Can you work these out from the drawing? Everything is in mm from the part's minimum corner. Coordinates: 2 decimals unless noted, no trailing zeros. Loops run counter-clockwise (first coordinate to the right, second up) from the corner with the lowest first, then second, coordinate; pieces in that order, holes last. Notation, with made-up numbers: (54, -27) - (63, -27) arc R30 ccw to (63, -1) - close; hole circle Ø5 at (39.5, -6.75). An arc over 180 degrees is marked (long way). One line per question, with ' | ' between items. Start each with the question number.
1. I want a section at D-D, the plane y = 40.5. Write out the boundary of the cut face in (x, z).
2. I want a section at C-C, the plane x = 60. Write out the boundary of the cut face in (y, z).
3. I want a section at B-B, the plane y = 10. Write out the boundary of the cut face in (x, z).
4. Please list where these lines run through material, in increasing order: L1, parallel to Y at x = 35, z = 0.85; L2, parallel to Y at x = 10, z = 2.05; L3, parallel to Y at x = 34, z = 0.95. Write a range as [from, to].
5. I'm going to push flat-ended pins straight in: P1, Ø3.5, axis at x = 35, y = 10, coming from the -Z side; P2, Ø2.5, axis at x = 60, y = 10, coming from the +Z side. Where does each tip first touch, or does it pass through?
6. I want a section at A-A, the plane x = 35. Write out the boundary of the cut face in (y, z).
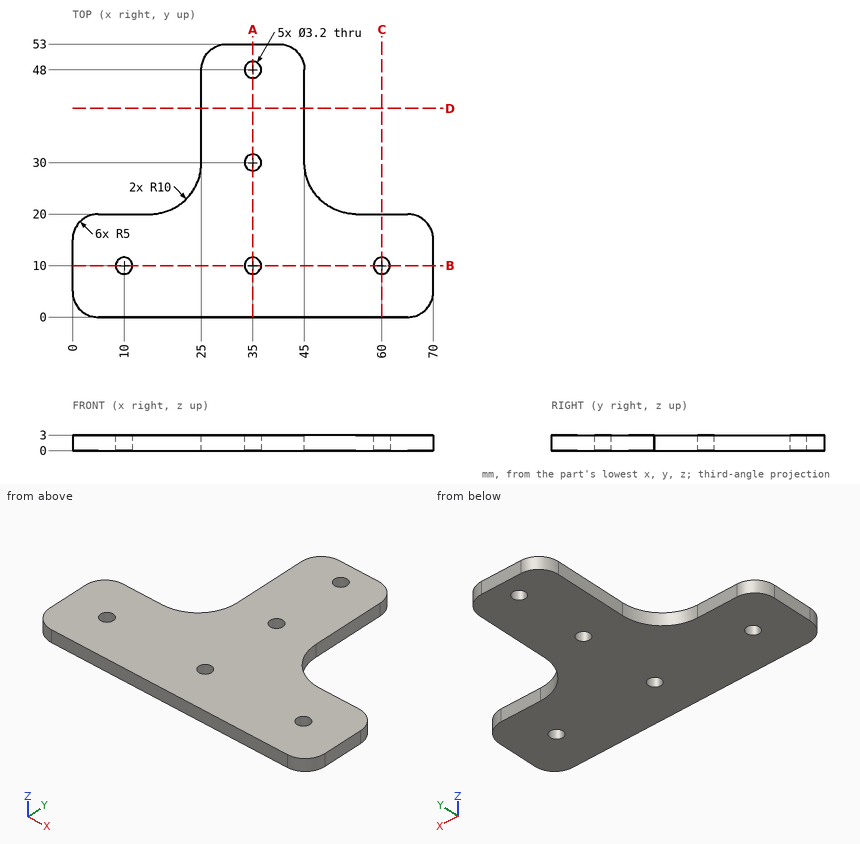
Results are:
1) outline: (25, 0) - (45, 0) - (45, 3) - (25, 3) - close
2) outline: (0, 0) - (8.4, 0) - (8.4, 3) - (0, 3) - close; (11.6, 0) - (20, 0) - (20, 3) - (11.6, 3) - close
3) outline: (0, 0) - (8.4, 0) - (8.4, 3) - (0, 3) - close; (11.6, 0) - (33.4, 0) - (33.4, 3) - (11.6, 3) - close; (36.6, 0) - (58.4, 0) - (58.4, 3) - (36.6, 3) - close; (61.6, 0) - (70, 0) - (70, 3) - (61.6, 3) - close
4) L1: y = [0, 8.4], [11.6, 28.4], [31.6, 46.4], [49.6, 53] | L2: y = [0, 8.4], [11.6, 20] | L3: y = [0, 8.75], [11.25, 28.75], [31.25, 46.75], [49.25, 53]
5) P1: stops at z = 0 | P2: passes through
6) outline: (0, 0) - (8.4, 0) - (8.4, 3) - (0, 3) - close; (11.6, 0) - (28.4, 0) - (28.4, 3) - (11.6, 3) - close; (31.6, 0) - (46.4, 0) - (46.4, 3) - (31.6, 3) - close; (49.6, 0) - (53, 0) - (53, 3) - (49.6, 3) - close
